from build123d import *

# Parameters (mm, degrees)
SKETCH_3_R      = 112.5
EXTRUDE_5_DEPTH = 5
EXTRUDE_1_REACH = 269.786
SKETCH_8_R      = 90.24770546
EXTRUDE_2_DEPTH = 10


with BuildPart() as part:
    # Sketch 3 → Extrude 5 (new body)
    with BuildSketch(Plane(origin=(0, 0, 0), x_dir=(-0.4082482904638631, -0.40824829046386274, -0.8164965809277263), z_dir=(0.5773502691896261, 0.5773502691896257, -0.5773502691896256))):
        with Locations(Location((0, 0, 0), (0, 0, 90))):
            Circle(SKETCH_3_R)
    extrude(amount=-EXTRUDE_5_DEPTH)

    # Extrude 1: up to this plane
    extrude_1_end = Plane(origin=(-2.886751346, -2.886751346, 2.886751346), z_dir=(0.5773502691896261, 0.5773502691896257, -0.5773502691896256))
    # Sketch 5 → Extrude 1 (add, up to the surface)
    with BuildSketch(Plane(origin=(0, -140, 0), x_dir=(1, 0, 0), z_dir=(0, 1, 0)), mode=Mode.PRIVATE) as extrude_1_sk1:
        Polygon((-37.158068765, 62.446542524), (-66.718597501, 32.886013788), (-66.718597501, -11.451165298), (-11.451165298, -66.718597501), (32.886013788, -66.718597501), (62.446542524, -37.158068765), (64.849763198, -13.752243339), (-13.752243339, 64.849763198), align=None)
    extrude_1_tool1 = split(extrude(extrude_1_sk1.sketch, amount=EXTRUDE_1_REACH, mode=Mode.PRIVATE), bisect_by=extrude_1_end, keep=Keep.BOTH, mode=Mode.PRIVATE)
    add(extrude_1_tool1.solids().sort_by_distance((-5.313204, -140, 5.313204))[0])

    # Sketch 8 → Extrude 2 (add)
    with BuildSketch(Plane(origin=(0, -140, 0), x_dir=(1, 0, 0), z_dir=(0, 1, 0))):
        with Locations(Location((0, 0, 0), (0, 0, 270))):
            Circle(SKETCH_8_R)
    extrude(amount=EXTRUDE_2_DEPTH)


solid = part.part
Here's how the part is built. I have some questions about the finished solid (model axes, mm). A direction names the side the tool comes from. Coordinates: 2 decimals unless noted, no trailing zeros.
Item 1: For faces 1 (the face through (47.459, -70.741, 52.145)), 2 (the face through (-66.719, -32, -11)), 3 (the face through (-51.731, -70.741, -47.873)), 4 (the face through (89.48, -135.07, -11.75)), 5 (the face through (21, -130, -41)), which set-ups out of +Z, -Z, +X, -X, +Y, -Y let a thin tool reach every point of the face, with its end or its side?
Result sheet:
face 1: +Z
face 2: +Z, -X
face 3: -X
face 4: -Y
face 5: none
Item 2: If we mould it in two halves opening along X, with no side actions, what happens to faces 6 (the face through (10, -32, 66.719)), 7 (the face through (63.63, -93.32, 25.62)), 8 (the face through (1.8, -0.5, 1.3))? For each: +X half, -X half, draft (parallel to the pull), parting line (faces both ways), or undercut.
Result sheet:
face 6: draft
face 7: undercut
face 8: +X half
Item 3: For P1, Ø1.5, axis at y = 41, z = 9.5, coming from the -X side; P2, Ø1.5, axis at x = -67, y = -72, coming from the +Z side; P3, Ø5, axis at x = -38, y = -101.5, coming from the -Z side, each with a flat end and sliding along its axis, tell me the tip position at first contact or that it passes through.
Result sheet:
P1: stops at x = -66.72
P2: stops at z = 11.92
P3: stops at z = -62.62
Item 4: I need wall thicknesses on line 1 (Y direction, x = -73.5, z = -28.5); line 2 (Y direction, x = 84, z = 26.5); line 3 (Y direction, x = -60, z = 39). Which ranges of each line are inside material? Lowest first, please.
Result sheet:
line 1: y = -140 to -130, 36.34 to 45
line 2: y = -140 to -130, -66.16 to -57.5
line 3: y = -140 to -130
